Source: CAD feature listing. Evaluate the final solid. Frame: model axes, mm. Face numbers are marked on the shaded views. A direction names the side the tool comes from. Coordinates: 2 decimals unless noted, no trailing zeros. Loops run counter-clockwise (first coordinate to the right, second up) from the corner with the lowest first, then second, coordinate; pieces in that order, holes last.
Item 1: Line query: probe 1 along X at (y, z) = (-6.25, 1.6); probe 2 along X at (y, z) = (8.75, 0.5); probe 3 along Y at (x, z) = (-8.25, 0.2). Output: solid intervals per line, ascending.
Item 2: Section query D-D, the plane y = 4. Return the cut outline in (x, z), then the cut area to 3 significant figures.
Item 3: Pin query (flat end, axial travel): pin 1 Ø1.6 at (y, z) = (-3.5, 1) entering from +X. Return the tip coordinate at first contact, or that it passes through.
Item 4: Reachability of the marked faces 1 and 2 from +Z, -Z, +X, -X, +Y, -Y: full face, straight path, thin tool, end or side. Return the list, or none.
Item 5: Section query A-A, the plane z = 0.8. State how many separate pieces and enclosed holes the cut face has, then the cut area to 3 significant figures.
Item 6: Pull-direction query (X, two-part tool) for the marked faces 3, 4 and 5; classes: +X half, -X half, draft (parallel to the pull), parting line (faces both ways), or undercut.
Item 7: Section query B-B, the plane y = 6.75. Return the cut outline in (x, z).
Item 8: Section query C-C, the plane y = -0.5. Return the cut outline in (x, z).
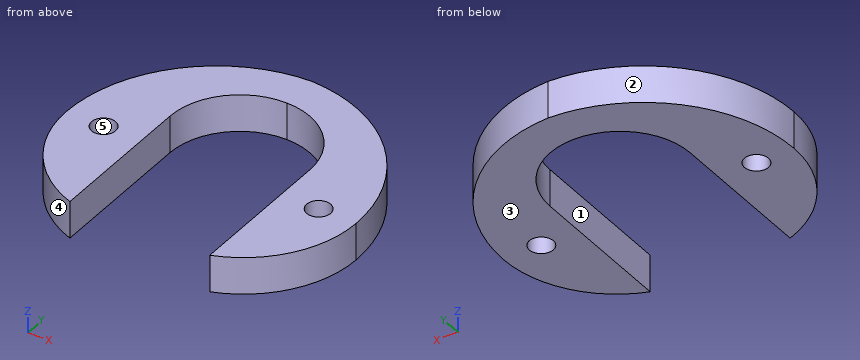
```python
from build123d import *

# Parameters (mm, degrees)
CROQUIS1_R              = 1.016
SALIENTE_EXTRUIR1_DEPTH = 3.1242


with BuildPart() as part:
    # Croquis1 → Saliente-Extruir1 (new body)
    with BuildSketch(Plane.XY):
        with BuildLine():
            Line((0, 9.525), (-2.7305, 9.525))
            ThreePointArc((-2.7305, 9.525), (-9.465692091, 6.735192091), (-12.2555, 0))
            ThreePointArc((-12.2555, 0), (-10.507629933, -5.499261314), (-5.9055, -8.980256121))
            Line((-5.9055, -8.980256121), (-5.9055, -3.6195))
            Line((-5.9055, -3.6195), (-5.9055, 3.6195))
            ThreePointArc((-5.9055, 3.6195), (-4.175819096, 7.795319096), (0, 9.525))
        make_face()
        with Locations((-9.0805, 0)):
            Circle(CROQUIS1_R, mode=Mode.SUBTRACT)
        with BuildLine():
            ThreePointArc((-12.2555, 0), (-9.465692091, 6.735192091), (-2.7305, 9.525))
            Line((-2.7305, 9.525), (0, 9.525))
            Line((0, 9.525), (2.7305, 9.525))
            ThreePointArc((2.7305, 9.525), (9.473939825, 6.726934244), (12.255471398, -0.023342399))
            ThreePointArc((12.255471398, -0.023342399), (8.702367859, 8.818284916), (0, 12.7))
            ThreePointArc((0, 12.7), (-8.691999868, 8.824501123), (-12.2555, 0))
        make_face()
        with BuildLine():
            Line((2.7305, 9.525), (0, 9.525))
            ThreePointArc((0, 9.525), (4.175819096, 7.795319096), (5.9055, 3.6195))
            Line((5.9055, 3.6195), (5.9055, -3.6195))
            Line((5.9055, -3.6195), (5.9055, -8.980256121))
            ThreePointArc((5.9055, -8.980256121), (10.50088572, -5.508786688), (12.255471398, -0.023342399))
            ThreePointArc((12.255471398, -0.023342399), (9.473939825, 6.726934244), (2.7305, 9.525))
        make_face()
        with Locations((9.0805, 0)):
            Circle(CROQUIS1_R, mode=Mode.SUBTRACT)
    extrude(amount=SALIENTE_EXTRUIR1_DEPTH)


solid = part.part
```
Verdict:
1. probe 1: x = -9.92 to -5.91, 5.91 to 9.92
1. probe 2: x = -8.76 to -2.92, 2.92 to 8.77
1. probe 3: y = -7.76 to -0.59, 0.59 to 9.26
2. outline: (-11.61, 0) - (-5.89, 0) - (-5.89, 3.12) - (-11.61, 3.12) - close; (5.89, 0) - (11.61, 0) - (11.61, 3.12) - (5.89, 3.12) - close
2. area: 35.7 mm2
3. pin 1: stops at x = 11.86
4. face 1: +Z, -Z, -Y
4. face 2: +Z, -Z, -X, +Y
5. separate pieces: 1
5. enclosed holes: 2
5. area: 221 mm2
6. face 3: draft
6. face 4: -X half
6. face 5: undercut
7. outline: (-10.31, 0) - (-5.01, 0) - (-5.01, 3.12) - (-10.31, 3.12) - close; (5.01, 0) - (10.32, 0) - (10.32, 3.12) - (5.01, 3.12) - close
8. outline: (-12.24, 0) - (-9.96, 0) - (-9.96, 3.12) - (-12.24, 3.12) - close; (-8.2, 0) - (-5.91, 0) - (-5.91, 3.12) - (-8.2, 3.12) - close; (5.91, 0) - (8.2, 0) - (8.2, 3.12) - (5.91, 3.12) - close; (9.96, 0) - (12.24, 0) - (12.24, 3.12) - (9.96, 3.12) - close
